```python
from build123d import *

# Parameters (mm, degrees)
BOSS_EXTRUDE2_DEPTH = 1
CIRPATTERN1_COUNT   = 6
SKETCH3_W           = 1.8
SKETCH3_H           = 7.2
CUT_EXTRUDE1_DEPTH  = 24.055801873
SKETCH4_R           = 1.2
CUT_EXTRUDE2_DEPTH  = 0.4
CIRPATTERN2_COUNT   = 6


with BuildPart() as part:
    # Sketch1 → Revolve1 (revolve)
    with BuildSketch(Plane.XY, mode=Mode.PRIVATE) as revolve1_sk:
        Polygon((15.8, 3.35), (15.8, 2.55), (15.3, 2.55), (15.3, 2.25), (0.5, 2.25), (0.5, 2.55), (0, 2.55), (0, 3.35), (6.3, 3.35), (6.3, 7.8), (1, 7.8), (1, 8.8), (7.2, 8.8), (7.2, 5.5), (9, 5.5), (9, 8.8), (10.8, 8.8), (10.8, 5.5), (12.8, 5.5), (12.8, 8.8), (14.8, 8.8), (14.8, 7.8), (13.8, 7.8), (13.8, 3.35), align=None)
    revolve(revolve1_sk.sketch.rotate(Axis((0, 0, 0), (1, 0, 0)), 90), axis=Axis((0, 0, 0), (1, 0, 0)))

    # Sketch2 → Boss-Extrude2 (add)
    with BuildSketch(Plane(origin=(13.8, 0, 0), x_dir=(0, 0, -1), z_dir=(1, 0, 0))):
        with BuildLine():
            Line((-1.5, 7.654410493), (-1.5, 2.99541316))
            ThreePointArc((-1.5, 2.99541316), (-1.012488161, 3.193331759), (-0.5, 3.312476415))
            Line((-0.5, 3.312476415), (-0.5, 7.783957862))
            ThreePointArc((-0.5, 7.783957862), (-1.002095619, 7.735360649), (-1.5, 7.654410493))
        make_face()
        with BuildLine():
            Line((0.5, 7.783957862), (0.5, 3.312476415))
            ThreePointArc((0.5, 3.312476415), (1.012469043, 3.193337821), (1.5, 2.99541316))
            Line((1.5, 2.99541316), (1.5, 7.654410493))
            ThreePointArc((1.5, 7.654410493), (1.002095619, 7.735360649), (0.5, 7.783957862))
        make_face()
    boss_extrude2 = extrude(amount=BOSS_EXTRUDE2_DEPTH)

    # CirPattern1: Boss-Extrude2 ×6 about axis
    cirpattern1_axis = Axis((0, 0, 0), (1, 0, 0))
    for i in range(1, CIRPATTERN1_COUNT):
        add(boss_extrude2.rotate(cirpattern1_axis, i * 360 / CIRPATTERN1_COUNT))

    # Sketch3 → Cut-Extrude1 (cut, through all)
    with BuildSketch(Plane(origin=(0, 5.5, 0), x_dir=(1, 0, 0), z_dir=(0, 1, 0))):
        with Locations((8.1, 0)):
            Rectangle(SKETCH3_W, SKETCH3_H)
    extrude(amount=-CUT_EXTRUDE1_DEPTH, mode=Mode.SUBTRACT)

    # Sketch4 → Cut-Extrude2 (cut)
    with BuildSketch(Plane.ZY.offset(-6.3)):
        with Locations((0, 6)):
            Circle(SKETCH4_R)
    cut_extrude2 = extrude(amount=-CUT_EXTRUDE2_DEPTH, mode=Mode.SUBTRACT)

    # CirPattern2: Cut-Extrude2 ×6 about axis
    cirpattern2_axis = Axis((0, 0, 0), (1, 0, 0))
    for i in range(1, CIRPATTERN2_COUNT):
        add(cut_extrude2.rotate(cirpattern2_axis, i * 360 / CIRPATTERN2_COUNT), mode=Mode.SUBTRACT)


solid = part.part
```
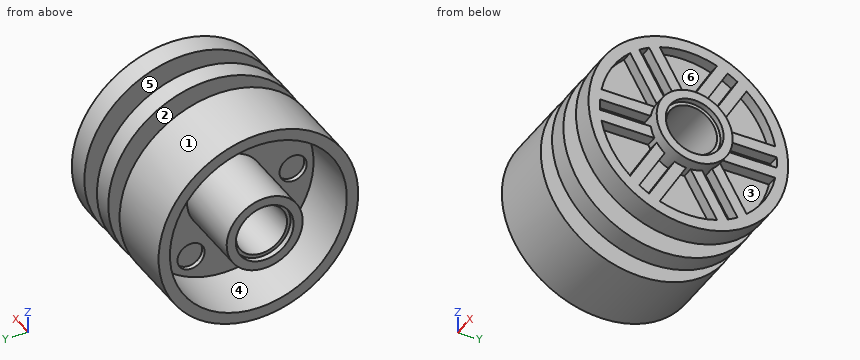
Here's how the part is built. I have some questions about the finished solid (model axes, mm). Face numbers are marked on the shaded views. A direction names the side the tool comes from. Coordinates: 2 decimals unless noted, no trailing zeros. Order: outer loops, then holes, each group sorted by start corner. A loop starts at its lowest first (then second) coordinate and runs counter-clockwise, first axis right, second up. Notation, with made-up numbers: M 35,37.25 L 87,37.25 A32 cw 87,76.25 Z; hole C 18,-9 d4. An arc over 180 degrees is marked long. Answer as a JSON object with one key per item and string values. Group by question number.
(1) If we mould it in two halves opening along Y, with no side actions, what happens to the marked faces 1, 2 and 3? For each: released by +Y, released by -Y, zero draft, split by the parting line, or undercut.
(2) Suppose I cut it at C-C, the plane z = 6.75. Please give me the cut outline in (x, y), then the cut area to 3 significant figures.
(3) Suppose I cut it at D-D, the plane x = 11.5. Please give me the cut outline in (y, z), then the cut area to 3 significant figures.
(4) Which directions (+Z, -Z, +X, -X, +Y, -Y) give clear straight access to the entire face, cutting with the end or side of a thin tool? Please do the marked faces 4, 5 and 6.
(5) I need wall thicknesses on probe 1 along Y at (x, z) = (6.4, 0); probe 2 along X at (y, z) = (4.75, 7.25); probe 3 along Y at (x, z) = (14.25, 0). Which ranges of each line are inside material? Lowest first, please.
(6) For pin 1 (1.2 mm diameter, centred on y = 3, z = -5.5, fed in from -X); pin 2 (0.5 mm diameter, centred on x = 14, y = 5.5, fed in from +Z); pin 3 (5 mm diameter, centred on x = 4, z = 6.5, fed in from +Y), each with a flat end and sliding along its axis, tell me the tip position at first contact or that it passes through.
(7) Suppose I cut it at A-A, the plane y = -6. State how many separate pieces and enclosed holes the cut face has, then the cut area to 3 significant figures.
Values found:
{
 "1": {"face 1": "split by the parting line", "face 2": "zero draft", "face 3": "undercut"},
 "2": {"outline": "M 1,-5.65 L 7.2,-5.65 L 7.2,5.65 L 1,5.65 L 1,3.91 L 6.3,3.91 L 6.3,-3.91 L 1,-3.91 Z; M 9,-5.65 L 10.8,-5.65 L 10.8,5.65 L 9,5.65 Z; M 12.8,-5.65 L 14.8,-5.65 L 14.8,-3.91 L 13.8,-3.91 L 13.8,-3.32 L 14.8,-3.32 L 14.8,-2.17 L 13.8,-2.17 L 13.8,2.17 L 14.8,2.17 L 14.8,3.32 L 13.8,3.32 L 13.8,3.91 L 14.8,3.91 L 14.8,5.65 L 12.8,5.65 Z", "area": "66.0 mm^2"},
 "3": {"outline": "C 0,0 d11; hole C 0,0 d4.5", "area": "79.1 mm^2"},
 "4": {"face 4": "-X", "face 5": "none", "face 6": "+X"},
 "5": {"probe 1": "y = -8.8 to -7.2, -4.8 to -2.25, 2.25 to 4.8, 7.2 to 8.8", "probe 2": "x = 1 to 7.2, 9 to 10.8, 12.8 to 14.8", "probe 3": "y = -8.8 to -7.8, -3.35 to -2.25, 2.25 to 3.35, 7.8 to 8.8"},
 "6": {"pin 1": "stops at x = 6.7", "pin 2": "stops at z = 7.06", "pin 3": "stops at y = 7.84"},
 "7": {"separate pieces": "3", "enclosed holes": "0", "area": "67.0 mm^2"}
}
